Build history of the part. All positions in model axes, mm. Coordinates: 2 decimals unless noted, no trailing zeros. Order: outer loops, then holes, each group sorted by start corner. A loop starts at its lowest first (then second) coordinate and runs counter-clockwise, first axis right, second up. Notation, with made-up numbers: M -17.5,-6 L 20.5,-6 A24 ccw 20.5,33 Z; hole C -18,65.25 d8. An arc over 180 degrees is marked long. Write item = value, one per line. Start each with the question number.
Q1. Band-saw the part on C-C on x = -64.5. Write the cut outline in (y, z).
Q2. Band-saw the part on A-A on y = 220. Write the cut outline in (x, z), plus the area to 3 significant figures.
Q3. Pull direction X, two halves, no side cores. Call faces 1 (the face through (-79.69, 169.89, 4.06)), 2 (the face through (65.396, 208.944, 3.944)), 3 (the face through (-3.255, 224.787, 4.056)): released by +X, released by -X, zero draft, split by the parting line, or undercut.
Q4. Drill centre lines: probe 1 along Y at (x, z) = (0, 3.75); probe 2 along X at (y, z) = (215, 7.25) (3 decimals); probe 3 along X at (y, z) = (207.5, 5.5). Where is each one in solid material? Low to high.
Q5. Band-saw the part on B-B on x = 0. Write the cut outline in (y, z), plus the area to 3 significant figures.
```python
from build123d import *

# Parameters (mm, degrees)
BOSS_EXTRUDE1_DEPTH = 8
SKETCH4_R           = 25
CUT_EXTRUDE1_DEPTH  = 8
FILLET2_R           = 20
FILLET4_R           = 20
FILLET5_R           = 10


with BuildPart() as part:
    # Sketch2 → Boss-Extrude1 (new body)
    with BuildSketch(Plane.XY):
        Polygon((-80, 0), (-80, 170), (-50, 250), (50, 250), (80, 170), (80, 0), align=None)
    extrude(amount=BOSS_EXTRUDE1_DEPTH)

    # Sketch4 → Cut-Extrude1 (cut)
    with BuildSketch(Plane.XY.offset(8)):
        with Locations((0, 200)):
            Circle(SKETCH4_R)
    extrude(amount=-CUT_EXTRUDE1_DEPTH, mode=Mode.SUBTRACT)

    # Fillet2
    fillet2_edges = [part.edges().sort_by_distance(p)[0] for p in [
        (-80, 170, 4),
    ]]
    fillet(fillet2_edges, radius=FILLET2_R)

    # Fillet4
    fillet4_edges = [part.edges().sort_by_distance(p)[0] for p in [
        (80, 170, 4),
    ]]
    fillet(fillet4_edges, radius=FILLET4_R)

    # Fillet5
    fillet5_edges = [part.edges().sort_by_distance(p)[0] for p in [
        (-50, 250, 4),
        (50, 250, 4),
    ]]
    fillet(fillet5_edges, radius=FILLET5_R)


solid = part.part
```
Recorded:
q1.outline = M 0,0 L 211.33,0 L 211.33,8 L 0,8 Z
q2.outline = M -61.25,0 L -15,0 L -15,8 L -61.25,8 Z; M 15,0 L 61.25,0 L 61.25,8 L 15,8 Z
q2.area = 740 mm2
q3.face_1 = released by -X
q3.face_2 = released by +X
q3.face_3 = undercut
q4.probe_1 = 0 to 175, 225 to 250
q4.probe_2 = -63.125 to -20, 20 to 63.125
q4.probe_3 = -65.94 to -23.85, 23.85 to 65.94
q5.outline = M 0,0 L 175,0 L 175,8 L 0,8 Z; M 225,0 L 250,0 L 250,8 L 225,8 Z
q5.area = 1,600 mm2
